Autodesk Inventor part; units mm, degrees
ref_plane "YZ Plane" through (0, 0, 0) normal (1, 0, 0) x (0, 1, 0)
ref_plane "XZ Plane" through (0, 0, 0) normal (0, 1, 0) x (-1, 0, 0)
ref_plane "XY Plane" through (0, 0, 0) normal (0, 0, 1) x (1, 0, 0)
sketch "Sketch1" plane through (0, 0, 0) normal (0, 0, 1) x (1, 0, 0)
  line L0 (-179.7163, 90.3709) -> (170.2837, 90.3709)
  line L1 (170.2837, 90.3709) -> (170.2837, -89.6291)
  line L2 (-179.7163, -89.6291) -> (-179.7163, 90.3709)
  line L3 (125.2837, -89.6291) -> (125.2837, 20.3709)
  line L4 (105.2837, 40.3709) -> (-114.7163, 40.3709)
  line L5 (-134.7163, 20.3709) -> (-134.7163, -89.6291)
  line L6 (170.2837, -89.6291) -> (125.2837, -89.6291)
  line L7 (-134.7163, -89.6291) -> (-179.7163, -89.6291)
  arc A0 (-114.7163, 40.3709) -> (-134.7163, 20.3709) centre (-114.7163, 20.3709) ccw
  arc A1 (125.2837, 20.3709) -> (105.2837, 40.3709) centre (105.2837, 20.3709) ccw
  point P0 (0, 0)
  dimension "d0" = 350
  dimension "d1" = 180
  dimension "d2" = 45
  dimension "d3" = 45
  dimension "d4" = 50
  dimension "d5" = 20
extrude "Extrusion1" add sketch "Sketch1" along normal blind 2
sketch "Sketch2" plane through (0, 0, 2) normal (0, 0, 1) x (1, 0, 0)
  line L0 (170.2837, 90.3709) -> (-179.7163, 90.3709)
  line L1 (-179.7163, 90.3709) -> (-129.7163, 90.3709)
  line L2 (-129.7163, 90.3709) -> (-129.7163, 85.3709)
  line L3 (-129.7163, 85.3709) -> (-179.7163, 85.3709)
  line L4 (-179.7163, 85.3709) -> (-179.7163, 90.3709)
  line L5 (-79.7163, 90.3709) -> (-29.7163, 90.3709)
  line L6 (-29.7163, 90.3709) -> (-29.7163, 85.3709)
  line L7 (-29.7163, 85.3709) -> (-79.7163, 85.3709)
  line L8 (-79.7163, 85.3709) -> (-79.7163, 90.3709)
  line L9 (20.2837, 90.3709) -> (70.2837, 90.3709)
  line L10 (70.2837, 90.3709) -> (70.2837, 85.3709)
  line L11 (70.2837, 85.3709) -> (20.2837, 85.3709)
  line L12 (20.2837, 85.3709) -> (20.2837, 90.3709)
  line L13 (170.2837, 90.3709) -> (120.2837, 90.3709)
  line L14 (120.2837, 90.3709) -> (120.2837, 85.3709)
  line L15 (120.2837, 85.3709) -> (170.2837, 85.3709)
  line L16 (170.2837, 85.3709) -> (170.2837, 90.3709)
  point P0 (0, 0)
  dimension "d8" = 50
  dimension "d9" = 50
  dimension "d10" = 50
  dimension "d11" = 50
  dimension "d12" = 50
  dimension "d13" = 50
  dimension "d14" = 50
  dimension "d15" = 5
extrude "Extrusion2" cut sketch "Sketch2" against normal blind 2
sketch "Sketch3" plane through (0, 0, 2) normal (0, 0, 1) x (1, 0, 0)
  line L0 (-179.7163, 85.3709) -> (-179.7163, -89.6291)
  line L1 (-179.7163, -53.6291) -> (-177.7163, -53.6291)
  line L2 (-177.7163, -53.6291) -> (-177.7163, -17.6291)
  line L3 (-177.7163, -17.6291) -> (-179.7163, -17.6291)
  line L4 (-179.7163, -17.6291) -> (-179.7163, -53.6291)
  line L5 (-179.7163, 18.3709) -> (-177.7163, 18.3709)
  line L6 (-177.7163, 18.3709) -> (-177.7163, 54.3709)
  line L7 (-177.7163, 54.3709) -> (-179.7163, 54.3709)
  line L8 (-179.7163, 54.3709) -> (-179.7163, 18.3709)
  line L9 (170.2837, -89.6291) -> (170.2837, 85.3709)
  line L10 (170.2837, -53.6291) -> (168.2837, -53.6291)
  line L11 (168.2837, -53.6291) -> (168.2837, -17.6291)
  line L12 (168.2837, -17.6291) -> (170.2837, -17.6291)
  line L13 (170.2837, -17.6291) -> (170.2837, -53.6291)
  line L14 (170.2837, 18.3709) -> (168.2837, 18.3709)
  line L15 (168.2837, 18.3709) -> (168.2837, 54.3709)
  line L16 (168.2837, 54.3709) -> (170.2837, 54.3709)
  line L17 (170.2837, 54.3709) -> (170.2837, 18.3709)
  line L18 (-179.7163, -89.6291) -> (-134.7163, -89.6291)
  line L19 (125.2837, -89.6291) -> (170.2837, -89.6291)
  point P0 (-177.7163, -35.6291)
  point P1 (-178.7163, -53.6291)
  point P2 (-178.7163, -17.6291)
  point P3 (-178.7163, 18.3709)
  point P4 (169.2837, -17.6291)
  point P5 (169.2837, 18.3709)
  point P6 (169.2837, -53.6291)
  dimension "d28" = 36
  dimension "d29" = 2
  dimension "d30" = 2
  dimension "d31" = 36
  dimension "d32" = 36
  dimension "d33" = 36
  dimension "d34" = 2
  dimension "d35" = 36
  dimension "d36" = 36
  dimension "d37" = 36
  dimension "d38" = 36
extrude "Extrusion3" cut sketch "Sketch3" against normal blind 2
properties part number "back"
The model under review builds one solid part; all positions refer to its coordinate system, in mm. A direction names the side the tool comes from. Round coordinates to 2 decimals unless told otherwise and drop trailing zeros. Order: outer loops, then holes, each group sorted by start corner. A loop starts at its lowest first (then second) coordinate and runs counter-clockwise, first axis right, second up. Notation, with made-up numbers: M 25,24 L 30,24 A25 ccw 30,63 Z; hole C 62,23.5 d1. An arc over 180 degrees is marked long. Use a Markdown table: item, result.
1) Insertion check: pin 1 (0.6 mm diameter, centred on y = 88.5, z = 1, fed in from +X); pin 2 (1 mm diameter, centred on x = -157.5, z = 1, fed in from +Y); pin 3 (0.6 mm diameter, centred on y = 39.5, z = 0.5, fed in from -X). Each pin has a flat end and moves straight along its axis. Give the tip position at first contact, or say it passes through.
Report:
| item | result |
|---|---|
| pin 1 | x = 120.28 |
| pin 2 | y = 85.37 |
| pin 3 | x = -177.72 |
2) Consider section B-B (y = -42). Write out the cut boundary in (x, z).
Report:
| item | result |
|---|---|
| outline | M -177.72,0 L -134.72,0 L -134.72,2 L -177.72,2 Z; M 125.28,0 L 168.28,0 L 168.28,2 L 125.28,2 Z |
3) Consider section C-C (x = -1.5). Write out the cut boundary in (y, z).
Report:
| item | result |
|---|---|
| outline | M 40.37,0 L 90.37,0 L 90.37,2 L 40.37,2 Z |
4) Consider section A-A (y = 6). Write out the cut boundary in (x, z).
Report:
| item | result |
|---|---|
| outline | M -179.72,0 L -134.72,0 L -134.72,2 L -179.72,2 Z; M 125.28,0 L 170.28,0 L 170.28,2 L 125.28,2 Z |
5) Wall thickness on line 1 along X through (y, z) = (-16, 0.3); line 2 along X through (y, z) = (-53, 0.75); line 3 along Y through (x, z) = (-62, 1.9): over which ranges is each line inside the solid? List them lowest first. Write a range as [from, to].
Report:
| item | result |
|---|---|
| line 1 | [-179.72, -134.72], [125.28, 170.28] |
| line 2 | [-177.72, -134.72], [125.28, 168.28] |
| line 3 | [40.37, 85.37] |
6) Tool access review of faces 3 (the face through (-7, 42, 0)), 4 (the face through (119.269, 34.668, 0.986)): name each direction out of +Z, -Z, +X, -X, +Y, -Y from which nothing blocks a thin tool from reaching the whole face with its end or side.
Report:
| item | result |
|---|---|
| face 3 | -Z, +X, -X, +Y, -Y |
| face 4 | +Z, -Z, -Y |
7) Consider section D-D (x = 43.5). Write out the cut boundary in (y, z).
Report:
| item | result |
|---|---|
| outline | M 40.37,0 L 85.37,0 L 85.37,2 L 40.37,2 Z |
8) Draft analysis for pull direction X (two halves, no side actions). For faces 1 (the face through (-129.01, 34.36, 0.99)), 2 (the face through (-7, 42, 2)), state which applies: released by +X, released by -X, zero draft, split by the parting line, or undercut.
Report:
| item | result |
|---|---|
| face 1 | undercut |
| face 2 | zero draft |
